Autodesk Inventor part; units mm, degrees
ref_plane "YZ Plane" through (0, 0, 0) normal (1, 0, 0) x (0, 1, 0)
ref_plane "XZ Plane" through (0, 0, 0) normal (0, 1, 0) x (-1, 0, 0)
ref_plane "XY Plane" through (0, 0, 0) normal (0, 0, 1) x (1, 0, 0)
sketch "Esboço1" plane through (0, 0, 0) normal (0, 0, 1) x (1, 0, 0)
  line L0 (0, 0) -> (101.5, 0)
  line L1 (0, 0) -> (-22.5, 22.5)
  line L2 (0, 0) -> (30, 0) construction
  line L3 (101.5, 0) -> (101.5, 22.5)
  line L4 (-22.5, 22.5) -> (-11.8934, 22.5)
  line L5 (-11.8934, 22.5) -> (-4.8223, 15.4289)
  line L6 (101.5, 22.5) -> (2.2487, 22.5)
  line L7 (-11.8934, 22.5) -> (-22.5, 22.5)
  line L8 (-22.5, 22.5) -> (-34.2669, 34.2669)
  line L9 (-4.8223, 15.4289) -> (-28.9636, 39.5702)
  line L10 (-4.8223, 15.4289) -> (2.2487, 22.5)
  dimension "d0" = 101.5
  dimension "d2" = 135
  dimension "d3" = 22.5
  dimension "d5" = 10
  dimension "d51" = 7.5
extrude "Extrusão1" add sketch "Esboço1" against normal blind 12
sketch "Esboço2" plane through (0, 0, 0) normal (0, 0, 1) x (1, 0, 0)
  line L0 (101.5, 22.5) -> (101.5, 0)
  line L1 (0, 0) -> (-22.5, 22.5)
  line L2 (2.2487, 22.5) -> (101.5, 22.5)
  line L3 (101.5, 22.5) -> (82.5, 22.5)
  point P0 (82.5, 11.25)
  point P1 (19.5, 11.25)
  point P2 (32.5, 13.45)
  point P3 (32.5, 9.05)
hole "Furo1" at (82.5, 11.25, 0) at (19.5, 11.25, 0) direction (0, 0, -1) diameter 6 end through all
hole "Furo2" at (32.5, 13.45, 0) direction (0, 0, -1) diameter 2 depth 7
hole "Furo3" at (32.5, 9.05, 0) direction (0, 0, -1) diameter 2 end through all
sketch "Esboço3" plane through (-4.8223, 15.4289, -12) normal (0.7071068, 0.7071068, 0) x (-0.7071068, 0.7071068, 0)
  line L0 (0, 12) -> (0, 0)
  line L1 (0, 6) -> (5, 6)
  point P0 (-14.3198, 12)
  dimension "d34" = 5
hole "Furo4" at (-8.3579, 18.9645, -6) direction (-0.7071068, -0.7071068, 0) diameter 6 end through all
sketch "Esboço4" plane through (2.2487, 22.5, 0) normal (0, 1, 0) x (1, 0, 0)
  line L0 (0, 0) -> (0, 12)
  line L1 (0, 12) -> (0, 5.7893)
  line L2 (99.2513, 12) -> (0, 12)
  line L3 (31.2513, 0) -> (29.2513, 0)
  line L4 (30.2513, 0) -> (30.2513, 6)
  point P0 (-2.2487, 0)
  dimension "d42" = 6.2107
hole "Furo5" at (32.5, 22.5, -6) direction (0, -1, 0) diameter 2 depth 18 counterbore diameter 6 counterbore depth 6
fillet "Arredondamento1" [suppressed]
properties part number "main_frame" material "Aluminum 6061-AHC"
Build history of the part. All positions in model axes, mm. A direction names the side the tool comes from. Give positions to 0.01 mm unless a question says otherwise; leave off trailing zeros. Order: outer loops, then holes, each group sorted by start corner. A loop starts at its lowest first (then second) coordinate and runs counter-clockwise, first axis right, second up. Notation, with made-up numbers: M 72,75.25 L 121,75.25 A23 ccw 121,105.25 Z; hole C 23.25,36 d5. An arc over 180 degrees is marked long. Put each result on its own line as item: value.
Item 1: Which spindle directions (+Z, -Z, +X, -X, +Y, -Y) get a long thin tool onto all of the face, cutting with end or side? Do faces 5 (the face through (-1.34, 18.91, -5.92)), 6 (the face through (32.2, 12.496, -3.042)), 7 (the face through (32.5, 15.3, -7)). Say none if no direction does.
Results are:
face 5: +Z, -Z, +Y
face 6: +Z
face 7: +Y
Item 2: Cut at D-D on z = -10.75. Write the cut outline in (x, y), then the cut area to 3 significant figures.
Results are:
outline: M -22.5,22.5 L 0,0 L 101.5,0 L 101.5,22.5 L 2.25,22.5 L -4.82,15.43 L -11.89,22.5 Z; hole C 19.5,11.25 d6; hole C 32.5,9.05 d2; hole C 82.5,11.25 d6
area: 2,430 mm2
Item 3: Drop flat-ended pins along their axis: pin 1 Ø0.6 at (x, y) = (32, 13.5) entering from +Z; pin 2 Ø1.2 at (x, z) = (32.5, -6) entering from +Y; pin 3 Ø2.5 at (x, z) = (32.5, -6) entering from +Y. Give the stop position or say it passes through.
Results are:
pin 1: z = -7
pin 2: y = 4.5
pin 3: y = 16.5
Item 4: Cut at B-B on y = 6.5. Write the cut outline in (x, z), then the cut area to 3 significant figures.
Results are:
outline: M -6.5,-12 L 101.5,-12 L 101.5,0 L -6.5,0 Z; hole C 32.5,-6 d2
area: 1,290 mm2
Item 5: Pull direction Z, two halves, no side cores. Call faces 1 (the face through (34, 16.5, -6)), 2 (the face through (39, 11, -12)), 3 (the face through (31.824, 6.238, -6.737)), 4 (the face through (50, 0, -6)): +Z half, -Z half, draft (parallel to the pull), parting line (faces both ways), or undercut.
Results are:
face 1: undercut
face 2: -Z half
face 3: undercut
face 4: draft
Item 6: Cut at A-A on x = 82.5. Write the cut outline in (y, z).
Results are:
outline: M 0,-12 L 8.25,-12 L 8.25,0 L 0,0 Z; M 14.25,-12 L 22.5,-12 L 22.5,0 L 14.25,0 Z
Item 7: Cut at C-C on z = -1.5. Write the cut outline in (x, y).
Results are:
outline: M -22.5,22.5 L 0,0 L 101.5,0 L 101.5,22.5 L 2.25,22.5 L -4.82,15.43 L -11.89,22.5 Z; hole C 19.5,11.25 d6; hole C 32.5,9.05 d2; hole C 32.5,13.45 d2; hole C 82.5,11.25 d6
Item 8: Wall check: probe 1 along Z at (x, y) = (32.5, 12.4); probe 2 along Z at (x, y) = (32.5, 20.9); probe 3 along X at (y, z) = (11.5, -8.75). Give the ranges that are in metal, low to high.
Results are:
probe 1: -12 to -7, -5 to 0
probe 2: -12 to -9, -3 to 0
probe 3: -11.5 to 16.51, 22.49 to 79.51, 85.49 to 101.5
